Geometry: final body of the model. Coordinates: model frame, mm. A direction names the side the tool comes from. Round coordinates to 2 decimals unless told otherwise and drop trailing zeros. Write each loop counter-clockwise with the first axis right and the second up, starting at its lowest first coordinate (ties: lowest second). Pieces come first, ordered by that corner, then holes. Notation, with made-up numbers: (22.25, 40) - (46.25, 40) arc R15 cw to (46.25, 56) - close; hole circle Ø11 at (68, -27.5). An arc over 180 degrees is marked (long way). Write each question's results on one line, items separated by ' | '.
from build123d import *

# Parameters (mm, degrees)
F0_R     = 4
F1_DEPTH = 3
F2_W     = 25
F2_H     = 50
F3_DEPTH = 28
F5_R     = 6
F6_DEPTH = 25
F7_W     = 19
F7_H     = 19
F8_DEPTH = 50
F4_R     = 4
F9_DEPTH = 50


with BuildPart() as f1:
    # F0 (on Top) → F1 (new body)
    with BuildSketch(Plane.XY):
        with BuildLine():
            Line((85, 7.5), (12.5, 7.5))
            Line((12.5, 7.5), (12.5, 37.5))
            Line((12.5, 37.5), (-12.5, 37.5))
            Line((-12.5, 37.5), (-12.5, -12.5))
            Line((-12.5, -12.5), (-11.479756, -12.5))
            Line((-11.479756, -12.5), (-47.281972, -134.636232))
            ThreePointArc((-47.281972, -134.636232), (-46.665777, -140.343315), (-42.194544, -143.943115))
            ThreePointArc((-42.194544, -143.943115), (-36.487461, -143.32692), (-32.887661, -138.855687))
            Line((-32.887661, -138.855687), (4.037017, -12.890273))
            ThreePointArc((4.037017, -12.890273), (4.097393, -12.694274), (4.163105, -12.5))
            Line((4.163105, -12.5), (12.5, -12.5))
            Line((12.5, -12.5), (12.5, -7.5))
            Line((12.5, -7.5), (85, -7.5))
            ThreePointArc((85, -7.5), (90.303301, -5.303301), (92.5, 0))
            ThreePointArc((92.5, 0), (90.303301, 5.303301), (85, 7.5))
        make_face()
        with Locations((-40.084816, -136.74596)):
            Circle(F0_R, mode=Mode.SUBTRACT)
        with Locations((85, 0)):
            Circle(F0_R, mode=Mode.SUBTRACT)
    extrude(amount=F1_DEPTH)

    # F2 (on face) → F3 (join)
    with BuildSketch(Plane.XY.offset(3)):
        with Locations((0, 12.5)):
            Rectangle(F2_W, F2_H)
    extrude(amount=-F3_DEPTH)

    # F5 (on face) → F6 (cut)
    with BuildSketch(Plane(origin=(-12.5, 0, 0), x_dir=(0, -1, 0), z_dir=(-1, 0, 0))):
        with Locations((-25, -12.5)):
            Circle(F5_R)
    extrude(amount=-F6_DEPTH, mode=Mode.SUBTRACT)

    # F7 (on face) → F8 (cut)
    with BuildSketch(Plane.XZ.offset(12.5)):
        with Locations((0, -12.5)):
            Rectangle(F7_W, F7_H)
    extrude(amount=-F8_DEPTH, mode=Mode.SUBTRACT)

    # F4 (on face) → F9 (join)
    with BuildSketch(Plane(origin=(0, 0, -25), x_dir=(1, 0, 0), z_dir=(0, 0, -1))):
        Circle(F4_R)
    extrude(amount=F9_DEPTH)


solid = f1.part
Q1. Section query A-A, the plane z = -12.5. Return loops of the section in (x, y).
Answer block:
outline: (-12.5, -12.5) - (-9.5, -12.5) - (-9.5, 19) - (-12.5, 19) - close; (-12.5, 31) - (-9.5, 31) - (-9.5, 37.5) - (-12.5, 37.5) - close; (9.5, -12.5) - (12.5, -12.5) - (12.5, 19) - (9.5, 19) - close; (9.5, 31) - (12.5, 31) - (12.5, 37.5) - (9.5, 37.5) - close
Q2. Ray query, line 1 along Z through (x, y) = (10, 25); line 2 along X through (y, z) = (30, -18); line 3 along Z through (x, y) = (79.5, 6.5). Return the intervals inside material, ascending.
Answer block:
line 1: -25 to -18.5, -6.5 to 3 | line 2: -12.5 to -9.5, 9.5 to 12.5 | line 3: 0 to 3
Q3. Pin query (flat end, axial travel): pin 1 (8.5 mm diameter, centred on y = 12, z = -15, fed in from -X); pin 2 (7.5 mm diameter, centred on x = 3, y = 10.5, fed in from -Z); pin 3 (3.5 mm diameter, centred on x = 39, z = 1.5, fed in from +Y). Return the tip coordinate at first contact, or that it passes through.
Answer block:
pin 1: x = -12.5 | pin 2: z = -25 | pin 3: y = 7.5
Q4. Section query C-C, the plane x = -6.5. Return loops of the section in (y, z), plus the area to 3 significant figures.
Answer block:
outline: (-48.84, 0) - (-12.5, 0) - (-12.5, -3) - (37.5, -3) - (37.5, 3) - (-48.84, 3) - close; (-12.5, -25) - (37.5, -25) - (37.5, -22) - (-12.5, -22) - close | area: 559 mm2
Q5. Section query D-D, the plane z = -35. Return loops of the section in (x, y).
Answer block:
outline: circle Ø8 at (0, 0)
Q6. Mould query, pull axis Z, two halves, no side actions, for faces 1 (the flat face through (9.5, 12, -13)), 2 (the cylindrical face through (-40.61, -132.78, 1.48)), 3 (the flat face through (52, 0, 0)), 4 (the flat face through (-4, -33, 3)). Classes: pulls with the +Z half, pulls with the -Z half, needs draft (parallel to the pull), parting line crosses it, or undercut.
Answer block:
face 1: undercut | face 2: needs draft | face 3: pulls with the -Z half | face 4: pulls with the +Z half
Q7. Section query B-B, the plane y = 25. Return loops of the section in (x, z), plus the area to 3 significant figures.
Answer block:
outline: (-12.5, -25) - (12.5, -25) - (12.5, -18.5) - (9.5, -18.5) - (9.5, -22) - (-9.5, -22) - (-9.5, -18.5) - (-12.5, -18.5) - close; (-12.5, -6.5) - (-9.5, -6.5) - (-9.5, -3) - (9.5, -3) - (9.5, -6.5) - (12.5, -6.5) - (12.5, 3) - (-12.5, 3) - close | area: 267 mm2
Q8. Access query for faces 5 (the cylindrical face through (81, 0, 1)), 6 (the flat face through (-12.5, 12, -11)), 7 (the flat face through (0, 12, -3)). Directions: +Z, -Z, +X, -X, +Y, -Y. A direction counts if a zero-diameter tool reaches every point of the face in a straight line with its end or side. Return the directions, or none.
Answer block:
face 5: +Z, -Z | face 6: +Z, -Z, -X, +Y | face 7: +Y, -Y
